Autodesk Inventor part; units mm, degrees
ref_plane "YZ Plane" through (0, 0, 0) normal (1, 0, 0) x (0, 1, 0)
ref_plane "XZ Plane" through (0, 0, 0) normal (0, 1, 0) x (-1, 0, 0)
ref_plane "XY Plane" through (0, 0, 0) normal (0, 0, 1) x (1, 0, 0)
sketch "Sketch1" plane through (0, 0, 0) normal (0, 0, 1) x (1, 0, 0)
  line L0 (14.5, -3) -> (-5.5, -3)
  line L1 (-5.5, -3) -> (-5.5, 3)
  line L2 (-5.5, 3) -> (14.5, 3)
  line L3 (14.5, 3) -> (14.5, 6)
  line L4 (11.5, 9) -> (-14.5, 9)
  line L5 (-14.5, 9) -> (-14.5, 0)
  line L6 (-14.5, 0) -> (-14.5, -9)
  line L7 (-14.5, -9) -> (11.5, -9)
  line L8 (14.5, -6) -> (14.5, -3)
  circle A0 centre (-0.5, 6) radius 1
  circle A1 centre (9.5, 6) radius 1
  circle A2 centre (-0.5, -6) radius 1
  circle A3 centre (9.5, -6) radius 1
  line L9 (14.5, -6) -> (11.5, -9)
  line L10 (11.5, 9) -> (14.5, 6)
  point P0 (0, 0)
extrude "Extrusion1" add sketch "Sketch1" along normal blind 3
sketch "Sketch2" plane through (0, 0, 3) normal (0, 0, 1) x (1, 0, 0)
  line L0 (-5.5, -3) -> (-5.5, 3)
  line L1 (-5.5, 3) -> (14.5, 3)
  line L2 (14.5, 3) -> (14.5, 6)
  line L3 (11.5, 9) -> (-14.5, 9)
  line L4 (-14.5, 9) -> (-14.5, -9)
  line L5 (-14.5, -9) -> (11.5, -9)
  line L6 (14.5, -6) -> (14.5, -3)
  line L7 (14.5, -3) -> (-5.5, -3)
  circle A0 centre (-0.5, 6) radius 1
  circle A1 centre (9.5, 6) radius 1
  circle A2 centre (-0.5, -6) radius 1
  circle A3 centre (9.5, -6) radius 1
  line L8 (14.5, 3) -> (14.5, 9)
  line L9 (14.5, -3) -> (14.5, 3)
  line L10 (11.5, -9) -> (14.5, -6)
  line L11 (14.5, 6) -> (11.5, 9)
  point P0 (0, 0)
extrude "Extrusion2" add sketch "Sketch2" along normal blind 5
chamfer "Chamfer1" distance 4 angle 45 1 edges at (-14.5, 0, 8)
fillet "Fillet1" radius 2 2 edges at (-12.5, 9, 6) (-12.5, -9, 6)
sketch "Sketch3" plane through (0, 0, 8) normal (0, 0, 1) x (1, 0, 0)
  line L0 (11.5, 9) -> (-7.6716, 9)
  ellipse E0 centre (-7.6716, 7) end of major axis (-10.5, 7) minor radius 2 (-7.6716, 9) -> (-10.5, 7) ccw
  line L1 (-10.5, -7) -> (-10.5, 7)
  ellipse E1 centre (-7.6716, -7) end of major axis (-10.5, -7) minor radius 2 (-10.5, -7) -> (-7.6716, -9) ccw
  line L2 (-7.6716, -9) -> (11.5, -9)
  line L3 (14.5, -6) -> (14.5, 6)
  circle A0 centre (-0.5, 6) radius 1
  circle A1 centre (9.5, 6) radius 1
  circle A2 centre (-0.5, -6) radius 1
  circle A3 centre (9.5, -6) radius 1
  line L4 (-3, 0) -> (3, 0) construction
  line L5 (-3, -2) -> (3, -2)
  line L6 (3, 2) -> (-3, 2)
  arc A4 (-3, 2) -> (-3, -2) centre (-3, 0) ccw
  arc A5 (3, -2) -> (3, 2) centre (3, 0) ccw
  line L7 (11.5, -9) -> (14.5, -6)
  line L8 (14.5, 6) -> (11.5, 9)
  point P0 (0, 0)
  dimension "d12" = 3
  dimension "d13" = 4
extrude "Extrusion3" cut sketch "Sketch3" against normal blind 5 contours A4 L6 A5 L5
chamfer "Chamfer3" distance 1 angle 45 4 edges at (5, 0, 8) (0, -2, 8) (-5, 0, 8) (0, 2, 8)
properties part number "end_tip_2"
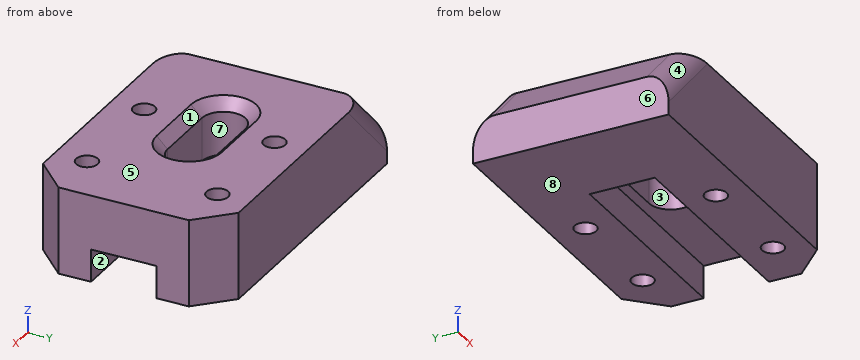
For this review, take the finished solid that the model builds, in its own axes (mm). Face numbers are marked on the shaded views. A direction names the side the tool comes from. Coordinates: 2 decimals unless noted, no trailing zeros. Write each loop counter-clockwise with the first axis right and the second up, starting at its lowest first coordinate (ties: lowest second). Pieces come first, ordered by that corner, then holes.
(1) Add section A-A on x = 2.25. Give the boundary of the cut face in (y, z), then the cut area to 3 significant figures.
(2) Tool access review of the marked faces 1, 2, 3, 4 and 5: name each direction out of +Z, -Z, +X, -X, +Y, -Y from which nothing blocks a thin tool from reaching the whole face with its end or side.
(3) The part is to be moulded in two halves that separate along X. For the marked faces 6, 7 and 8, say which applies: +X half, -X half, draft (parallel to the pull), parting line (faces both ways), or undercut.
(4) Wall thickness on probe 1 along Y at (x, z) = (-0.5, 4); probe 2 along Y at (x, z) = (9.5, 4.5); probe 3 along Y at (x, z) = (-0.5, 2.25): over which ranges is each line inside the solid? List them lowest first.
(5) For pin 1 Ø1.2 at (x, y) = (9.5, 6) entering from +Z; pin 2 Ø2.5 at (y, z) = (1, 1.5) entering from +X; pin 3 Ø1.8 at (x, y) = (9, -1) entering from -Z, all flat-tipped, find the tip position at first contact; note any pin that passes through.
(6) Add section D-D on y = -4. Give the boundary of the cut face in (x, z), then the cut area to 3 significant figures.
(7) Add section C-C on x = 9.5. Give the boundary of the cut face in (y, z).
(8) Add section B-B on y = 0. Give the boundary of the cut face in (x, z), then the cut area to 3 significant figures.
Answer sheet:
1. outline: (-9, 0) - (-3, 0) - (-3, 3) - (-2, 3) - (-2, 7) - (-3, 8) - (-9, 8) - close; (2, 3) - (3, 3) - (3, 0) - (9, 0) - (9, 8) - (3, 8) - (2, 7) - close
1. area: 105 mm2
2. face 1: +Z
2. face 2: -Z, +X
2. face 3: +Z, -Z
2. face 4: +Z, -X, -Y
2. face 5: +Z, +X, -X, +Y, -Y
3. face 6: -X half
3. face 7: undercut
3. face 8: draft
4. probe 1: y = -9 to -7, -5 to -2, 2 to 5, 7 to 9
4. probe 2: y = -9 to -7, -5 to 5, 7 to 9
4. probe 3: y = -9 to -7, -5 to -3, 3 to 5, 7 to 9
5. pin 1: passes through
5. pin 2: stops at x = -5.5
5. pin 3: stops at z = 3
6. outline: (-14.5, 0) - (14.5, 0) - (14.5, 8) - (-10.5, 8) - (-14.5, 4) - close
6. area: 224 mm2
7. outline: (-9, 0) - (-7, 0) - (-7, 8) - (-9, 8) - close; (-5, 0) - (-3, 0) - (-3, 3) - (3, 3) - (3, 0) - (5, 0) - (5, 8) - (-5, 8) - close; (7, 0) - (9, 0) - (9, 8) - (7, 8) - close
8. outline: (-14.5, 0) - (-5.5, 0) - (-5.5, 3) - (-5, 3) - (-5, 7) - (-6, 8) - (-10.5, 8) - (-14.5, 4) - close; (5, 3) - (14.5, 3) - (14.5, 8) - (6, 8) - (5, 7) - close
8. area: 113 mm2
